```python
from build123d import *

# Parameters (mm, degrees)
RESSALTO_EXTRUS_O1_DEPTH = 6
ESBO_O2_R                = 2.38125
CORTE_EXTRUS_O1_DEPTH    = 75.491610266


with BuildPart() as part:
    # Esboço1 → Ressalto-extrusão1 (new body)
    with BuildSketch(Plane.XY):
        with BuildLine():
            ThreePointArc((24.993351584, -7.164661654), (0, 26), (-24.993351584, -7.164661654))
            ThreePointArc((-24.993351584, -7.164661654), (-24.67461016, -12.336769329), (-26.566359725, -17.161038961))
            ThreePointArc((-26.566359725, -17.161038961), (0, -67), (26.566359725, -17.161038961))
            ThreePointArc((26.566359725, -17.161038961), (24.67461016, -12.336769329), (24.993351584, -7.164661654))
        make_face()
    extrude(amount=RESSALTO_EXTRUS_O1_DEPTH)

    # Esboço2 → Corte-extrusão1 (cut, through all)
    with BuildSketch(Plane.XY.offset(6)):
        with Locations((-14.849242405, 14.849242405)):
            Circle(ESBO_O2_R)
        with Locations((-19.528744622, -10.471428571)):
            Circle(ESBO_O2_R)
        with Locations((14.849242405, 14.849242405)):
            Circle(ESBO_O2_R)
        with Locations((19.528744622, -10.471428571)):
            Circle(ESBO_O2_R)
        with Locations((-26.07999731, -41.988114218)):
            Circle(ESBO_O2_R)
        with Locations((0, -62)):
            Circle(ESBO_O2_R)
        with Locations((26.07999731, -41.988114218)):
            Circle(ESBO_O2_R)
    extrude(amount=-CORTE_EXTRUS_O1_DEPTH, mode=Mode.SUBTRACT)


solid = part.part
```
The listing builds one solid part. Answer for the finished solid, in the listing's coordinates (mm). Round coordinates to 2 decimals unless told otherwise and drop trailing zeros. Order: outer loops, then holes, each group sorted by start corner. A loop starts at its lowest first (then second) coordinate and runs counter-clockwise, first axis right, second up. Notation, with made-up numbers: (-34.5, 50) - (10.5, 50) arc R18 cw to (10.5, 66) - close; hole circle Ø10 at (-8, 73). An arc over 180 degrees is marked (long way). Put each result on its own line as item: value. Start each with the question number.
(1) Find section B-B (z = 4.5). Give the vertices of the cut face in (x, y).
(2) Determine the mould class of faces 1 (the cylindrical face through (27.18, -44.1, 3.04)), 2 (the cylindrical face through (0.67, 25.99, 2.96)), 3 (the flat face through (0, -20, 6)) for opening direction X: released by +X, released by -X, zero draft, split by the parting line, or undercut.
(3) Given P1, Ø1, axis at x = 18, z = 1, coming from the +Y side; P2, Ø1.5, axis at y = -17.5, z = 5, coming from the -X side; P3, Ø1.5, axis at x = 15.5, z = 3.5, coming from the +Y side, each flat-ended and moving along its own axis, determine where each tip first touches the part or whether it passes through.
(4) Find section A-A (x = 0). Give the vertices of the cut face in (y, z), plus the area to 3 significant figures.
(5) Find section D-D (y = 0). Give the vertices of the cut face in (x, z).
(6) Straight lines are drawn through the part: probe 1 along X at (y, z) = (-56.5, 1.95); probe 2 along Y at (x, z) = (20, 2.1); probe 3 along Y at (x, z) = (-27.5, 3.75). For each, find the intervals that lie inside material, in ascending order. Write a range as from..to.
(7) Find section C-C (y = -62). Give the vertices of the cut face in (x, z), plus the area to 3 significant figures.
Reply:
1. outline: (-26.57, -17.16) arc R32 ccw (long way) to (26.57, -17.16) arc R12 cw to (24.99, -7.16) arc R26 ccw (long way) to (-24.99, -7.16) arc R12 cw to start; hole circle Ø4.76 at (-26.08, -41.99); hole circle Ø4.76 at (-19.53, -10.47); hole circle Ø4.76 at (-14.85, 14.85); hole circle Ø4.76 at (0, -62); hole circle Ø4.76 at (14.85, 14.85); hole circle Ø4.76 at (19.53, -10.47); hole circle Ø4.76 at (26.08, -41.99)
2. face 1: undercut
2. face 2: split by the parting line
2. face 3: zero draft
3. P1: y = 19.23
3. P2: x = -27.27
3. P3: y = 21.41
4. outline: (-67, 0) - (-64.38, 0) - (-64.38, 6) - (-67, 6) - close; (-59.62, 0) - (26, 0) - (26, 6) - (-59.62, 6) - close
4. area: 529 mm^2
5. outline: (-26, 0) - (26, 0) - (26, 6) - (-26, 6) - close
6. probe 1: -23.7..23.7
6. probe 2: -59.98..-12.81, -8.14..16.61
6. probe 3: -51.36..-43.9, -40.08..-18.64
7. outline: (-17.18, 0) - (-2.38, 0) - (-2.38, 6) - (-17.18, 6) - close; (2.38, 0) - (17.18, 0) - (17.18, 6) - (2.38, 6) - close
7. area: 178 mm^2
